Can you work these out from the model? Positions are in its coordinate system, mm. Give positions to 0.01 mm unless a question says otherwise; leave off trailing zeros. Write each loop counter-clockwise with the first axis right and the second up, starting at its lowest first coordinate (ties: lowest second). Pieces come first, ordered by that corner, then holes. Notation, with made-up numbers: M -17.5,-4 L 10.5,-4 A31 ccw 10.5,23 Z; hole C -1.75,-13.75 d1. An arc over 180 degrees is marked long. Write each question's results on one line, items separated by ' | '.
from build123d import *

# Parameters (mm, degrees)
BOSS_EXTRUDE1_DEPTH      = 8.98
BOSS_EXTRUDE1_DEPTH_BACK = 8.98


with BuildPart() as part:
    # Sketch1 → Boss-Extrude1 (new, two sides: drawn at the far end of the back side and taken through both)
    with BuildSketch(Plane.XY.offset(-BOSS_EXTRUDE1_DEPTH_BACK)):
        Polygon((3.175, -1.833087105), (3.175, 1.833087105), (0, 3.666174209), (-3.175, 1.833087105), (-3.175, -1.833087105), (0, -3.666174209), align=None)
    extrude(amount=BOSS_EXTRUDE1_DEPTH + BOSS_EXTRUDE1_DEPTH_BACK)

    # Sketch3 → Cut-Revolve2 (revolve, cut)
    with BuildSketch(Plane(origin=(0, 0, 0), x_dir=(0, 0, -1), z_dir=(1, 0, 0)), mode=Mode.PRIVATE) as cut_revolve2_sk:
        Polygon((-7.98, 3.666174209), (-8.98, 2.666174209), (-8.98, 3.666174209), align=None)
    cut_revolve2 = revolve(cut_revolve2_sk.sketch.rotate(Axis((0, 0, -0.635), (0, 0, 1)), 90), axis=Axis((0, 0, -0.635), (0, 0, 1)), mode=Mode.SUBTRACT)

    # Mirror1: Cut-Revolve2 across plane
    add(cut_revolve2.mirror(Plane.XY), mode=Mode.SUBTRACT)

    # Sketch4 → CSK for _1 Flat Head Machine Screw _100 (revolve, cut)
    with BuildSketch(Plane(origin=(0, 0, 8.98), x_dir=(0, -1, 0), z_dir=(1, 0, 0))):
        Polygon((0, 0), (0, 17.96), (1.6637, 17.96), (1.4, 17.6963), (1.4, 0.381119052), (1.8542, 0), align=None)
    revolve(axis=Axis((0, 0, 15.33), (0, 0, -1)), mode=Mode.SUBTRACT)


solid = part.part
Item 1: If I drill on line 1 (X direction, y = 0, z = -4.5) (3 decimals); line 2 (Y direction, x = 1, z = 2.5); line 3 (X direction, y = -0.75, z = -2.75) (3 decimals), over which ranges is the centre line in solid material (lowest first)? Write a range as from..to.
Geometry says:
line 1: x = -3.175..-1.4, 1.4..3.175 | line 2: y = -3.09..-0.98, 0.98..3.09 | line 3: x = -3.175..-1.182, 1.182..3.175
Item 2: Thinking about a two-plate mould opening in Y: for faces 1 (the face through (-0.06, 1.4, 0.06)), 2 (the face through (1.57, -2.76, -0.12)), 3 (the face through (1.61, 2.737, -0.119)), 4 (the face through (3.175, 0, 0)), which applies, +Y half, -Y half, draft (parallel to the pull), parting line (faces both ways), or undercut?
Geometry says:
face 1: undercut | face 2: -Y half | face 3: +Y half | face 4: draft
Item 3: I want a section at A-A, the plane y = 0. Please give me the cut outline in (x, z) (3 decimals), and give its area (3 significant figures).
Geometry says:
outline: M -3.175,-8.471 L -2.666,-8.98 L -1.664,-8.98 L -1.4,-8.716 L -1.4,8.599 L -1.854,8.98 L -2.666,8.98 L -3.175,8.471 Z; M 1.4,-8.716 L 1.664,-8.98 L 2.666,-8.98 L 3.175,-8.471 L 3.175,8.471 L 2.666,8.98 L 1.854,8.98 L 1.4,8.599 Z | area: 63.0 mm2
Item 4: I want a section at B-B, the plane z = 4.5. Please give me the cut outline in (x, y) (3 decimals).
Geometry says:
outline: M -3.175,-1.833 L 0,-3.666 L 3.175,-1.833 L 3.175,1.833 L 0,3.666 L -3.175,1.833 Z; hole C 0,0 d2.8
